The figure shows three views and two pictorial views of one solid part (mm, origin at its lowest corner). Answer the questions. Coordinates: 2 decimals unless noted, no trailing zeros. Order: outer loops, then holes, each group sorted by start corner. A loop starts at its lowest first (then second) coordinate and runs counter-clockwise, first axis right, second up. Notation, with made-up numbers: (-20.5, 78) - (-16.5, 78) arc R14 ccw to (-16.5, 100) - close; hole circle Ø10 at (0, 24). An arc over 180 degrees is marked (long way). Use one line per item in the form item = value.
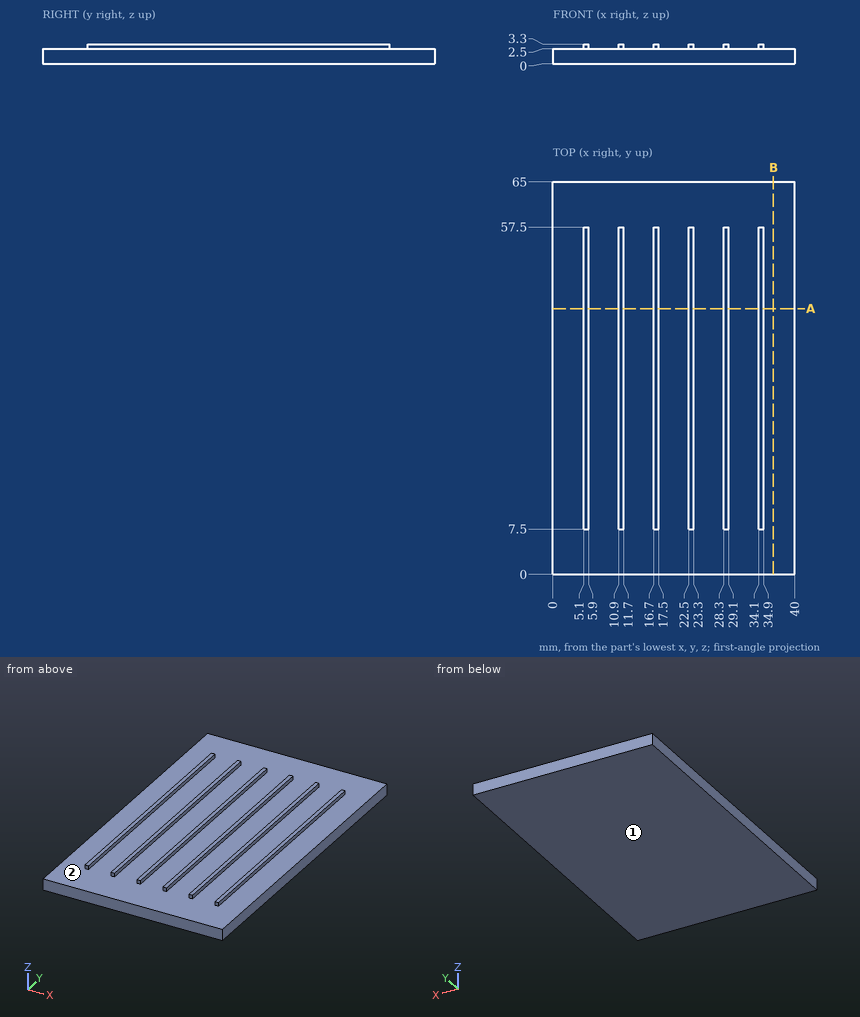
(1) Given pin 1 Ø0.9 at (x, z) = (5.5, 3) entering from +Y; pin 2 Ø0.6 at (y, z) = (36, 3) entering from -X; pin 3 Ø0.9 at (x, z) = (34.5, 3) entering from -Y; pin 4 Ø1.5 at (x, z) = (33.5, 1.5) entering from -Y, each flat-ended and moving along its own axis, determine where each tip first touches the part or whether it passes through.
Answer list:
pin_1 = 57.5
pin_2 = 5.1
pin_3 = 7.5
pin_4 = 0
(2) Section B-B, the plane x = 36.5 is taken. Write down the section's boundary in (y, z).
Answer list:
outline = (0, 0) - (65, 0) - (65, 2.5) - (0, 2.5) - close
(3) A straight line is drawn through the part: L1, parallel to Z at x = 18, y = 35.5. Find the intervals that lie inside material, in ascending order.
Answer list:
L1 = 0 to 2.5
(4) Section A-A, the plane y = 44 is taken. Write down the section's boundary in (x, z), then the cut area to 3 significant figures.
Answer list:
outline = (0, 0) - (40, 0) - (40, 2.5) - (34.9, 2.5) - (34.9, 3.3) - (34.1, 3.3) - (34.1, 2.5) - (29.1, 2.5) - (29.1, 3.3) - (28.3, 3.3) - (28.3, 2.5) - (23.3, 2.5) - (23.3, 3.3) - (22.5, 3.3) - (22.5, 2.5) - (17.5, 2.5) - (17.5, 3.3) - (16.7, 3.3) - (16.7, 2.5) - (11.7, 2.5) - (11.7, 3.3) - (10.9, 3.3) - (10.9, 2.5) - (5.9, 2.5) - (5.9, 3.3) - (5.1, 3.3) - (5.1, 2.5) - (0, 2.5) - close
area = 104 mm2
(5) The mould has two halves that part along X. Classify the marked faces 1 and 2: +X half, -X half, draft (parallel to the pull), parting line (faces both ways), or undercut.
Answer list:
face_1 = draft
face_2 = undercut
